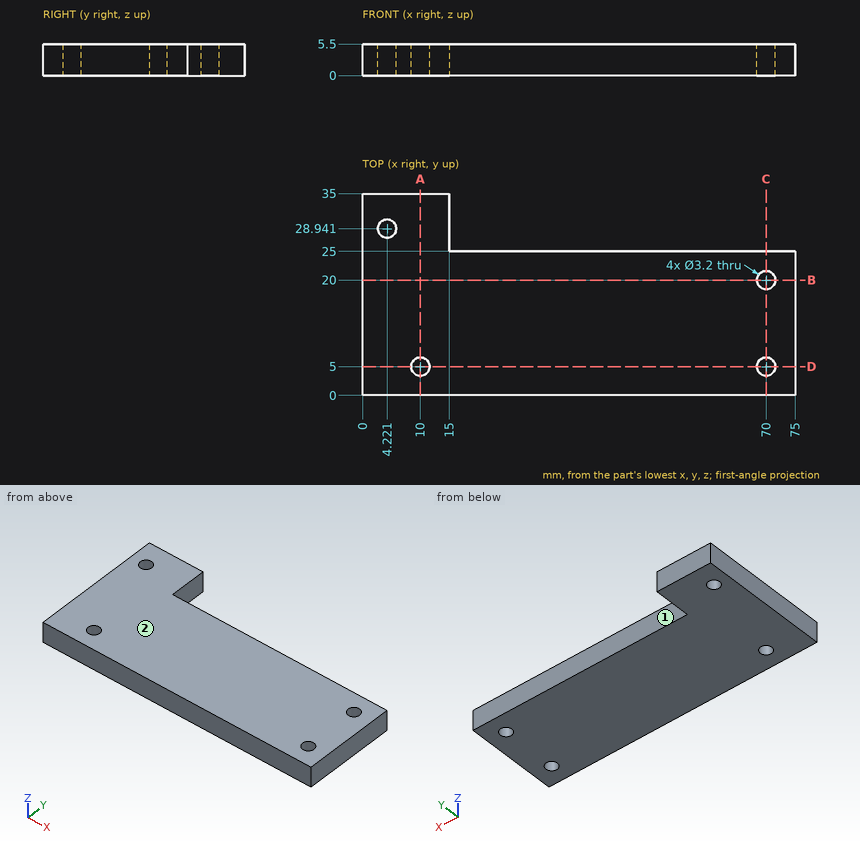
The drawing under review shows one solid part. Ordinate dimensions are in mm from its lowest x, y, z. A direction names the side the tool comes from. Give positions to 0.01 mm unless a question says otherwise; leave off trailing zeros. Write each loop counter-clockwise with the first axis right and the second up, starting at its lowest first coordinate (ties: lowest second). Pieces come first, ordered by that corner, then holes. Notation, with made-up numbers: (11.5, -18) - (54.5, -18) arc R24 ccw to (54.5, 18) - close; hole circle Ø8 at (48, -7.75). An arc over 180 degrees is marked (long way). Answer in a Markdown table with one row per item. Add a question column.
1. Insertion check: P1, Ø5, axis at x = 39, y = 29.5, coming from the -Z side; P2, Ø1.6, axis at y = 28, z = 3, coming from the +X side; P3, Ø3, axis at x = 41.5, z = 4.5, coming from the +Y side. Each pin has a flat end and moves straight along its axis. Give the tip position at first contact, or say it passes through.
2. We need section A-A on x = 10. Write out the cut boundary in (y, z), then the cut area to 3 significant figures.
3. Wall thickness on line 1 along X through (y, z) = (5, 4.1); line 2 along Y through (x, z) = (10, 3.85); line 3 along Y through (x, z) = (70, 3.45): over which ranges is each line inside the solid? List them lowest first. Write a range as [from, to].
4. Tool access review of the marked faces 1 and 2: name each direction out of +Z, -Z, +X, -X, +Y, -Y from which nothing blocks a thin tool from reaching the whole face with its end or side.
5. We need section D-D on y = 5. Write out the cut boundary in (x, z), then the cut area to 3 significant figures.
6. We need section C-C on x = 70. Write out the cut boundary in (y, z).
7. We need section B-B on y = 20. Write out the cut boundary in (x, z).
Ans:
| question | item | result |
|---|---|---|
| 1 | P1 | passes through |
| 1 | P2 | stops at x = 15 |
| 1 | P3 | stops at y = 25 |
| 2 | outline | (0, 0) - (3.4, 0) - (3.4, 5.5) - (0, 5.5) - close; (6.6, 0) - (35, 0) - (35, 5.5) - (6.6, 5.5) - close |
| 2 | area | 175 mm^2 |
| 3 | line 1 | x = [0, 8.4], [11.6, 68.4], [71.6, 75] |
| 3 | line 2 | y = [0, 3.4], [6.6, 35] |
| 3 | line 3 | y = [0, 3.4], [6.6, 18.4], [21.6, 25] |
| 4 | face 1 | +Z, -Z, +X, +Y |
| 4 | face 2 | +Z, +X, -X, +Y, -Y |
| 5 | outline | (0, 0) - (8.4, 0) - (8.4, 5.5) - (0, 5.5) - close; (11.6, 0) - (68.4, 0) - (68.4, 5.5) - (11.6, 5.5) - close; (71.6, 0) - (75, 0) - (75, 5.5) - (71.6, 5.5) - close |
| 5 | area | 377 mm^2 |
| 6 | outline | (0, 0) - (3.4, 0) - (3.4, 5.5) - (0, 5.5) - close; (6.6, 0) - (18.4, 0) - (18.4, 5.5) - (6.6, 5.5) - close; (21.6, 0) - (25, 0) - (25, 5.5) - (21.6, 5.5) - close |
| 7 | outline | (0, 0) - (68.4, 0) - (68.4, 5.5) - (0, 5.5) - close; (71.6, 0) - (75, 0) - (75, 5.5) - (71.6, 5.5) - close |
